For this review, take the finished solid that the model builds, in its own axes (mm). A direction names the side the tool comes from. Coordinates: 2 decimals unless noted, no trailing zeros. Order: outer loops, then holes, each group sorted by start corner. A loop starts at its lowest first (then second) coordinate and runs counter-clockwise, first axis right, second up. Notation, with made-up numbers: (89, 19) -> (99, 19) arc R8 ccw to (99, 26) -> close; hole circle Ø5 at (-29, 45). An arc over 180 degrees is marked (long way). Answer as a JSON object with one key per item and string values. Group by question number.
1) Add section B-B, the plane y = -1.5. Write out the cut boundary in (x, z), then the cut area to 3 significant figures.
2) For pin 1 (5 mm diameter, centred on x = 12, z = 1, fed in from -Y); pin 2 (1.5 mm diameter, centred on x = -4, z = 7.5, fed in from +Y); pin 3 (0.7 mm diameter, centred on y = -6, z = 2.5, fed in from +X); pin 4 (2 mm diameter, centred on x = 6.5, y = 0.5, fed in from -Z), all flat-tipped, find the tip position at first contact; note any pin that passes through.
3) Add section D-D, the plane x = 5.5. Write out the cut boundary in (y, z).
4) Add section A-A, the plane z = 2.75. Write out the cut boundary in (x, y), then the cut area to 3 significant figures.
5) Wall thickness on L1, parallel to Y at x = 5.5, z = 5.75; L2, parallel to Y at x = 0, z = 3.5; L3, parallel to X at y = 1, z = 3.75: over which ranges is each line inside the solid? List them lowest first.
6) Machinability: for faces 5 (the flat face through (-7.933, 2, 4)), 6 (the flat face through (6, -3.137, 4)), which of the approach directions +Z, -Z, +X, -X, +Y, -Y give a long, thin tool a straight path to every point of the face, cutting with its end or side? Answer none if there is none.
7) Draft analysis for pull direction X (two halves, no side actions). For faces 1 (the cylindrical face through (-0.54, -2.44, 4.44)), 2 (the flat face through (-5, -7, 4)), 3 (the flat face through (12.67, 7.07, 4.44)), 4 (the flat face through (2, 5.957, 4)), state which applies: +X half, -X half, draft (parallel to the pull), parting line (faces both ways), or undercut.
8) Add section C-C, the plane x = 0. Write out the cut boundary in (y, z), then the cut area to 3 significant figures.
from build123d import *

# Parameters (mm, degrees)
SKETCH_1_R      = 2.5
EXTRUDE_1_DEPTH = 9


with BuildPart() as part:
    # 스케치1 → 보스-돌출1 (new body)
    with BuildSketch(Plane.XY):
        with BuildLine():
            Line((-7.933325128, 1.188242905), (-5, -2.066412243))
            Line((-5, -2.066412243), (-5, -11.820871263))
            Line((-5, -11.820871263), (-3.253479839, -11.820871263))
            Line((-3.253479839, -11.820871263), (1.87605446, -7.031414053))
            Line((1.87605446, -7.031414053), (1.87605446, -4.634697365))
            ThreePointArc((1.87605446, -4.634697365), (2.980195691, -4.014776911), (3.893195608, -3.13736003))
            Line((3.893195608, -3.13736003), (9.172978659, -3.13736003))
            Line((9.172978659, -3.13736003), (14.557074242, 2.286312605))
            Line((14.557074242, 2.286312605), (14.557074242, 5.198022376))
            Line((14.557074242, 5.198022376), (10.725649804, 9.001488547))
            Line((10.725649804, 9.001488547), (6.528593017, 9.001488547))
            Line((6.528593017, 9.001488547), (6.037882178, 5.957406269))
            Line((6.037882178, 5.957406269), (-1.376355668, 5.957406269))
            Line((-1.376355668, 5.957406269), (-7.933325128, 2.286312605))
            Line((-7.933325128, 2.286312605), (-7.933325128, 1.188242905))
        make_face()
        Circle(SKETCH_1_R, mode=Mode.SUBTRACT)
    extrude(amount=EXTRUDE_1_DEPTH)


solid = part.part
Output values:
{
 "1": {"outline": "(-5.51, 0) -> (-2, 0) -> (-2, 9) -> (-5.51, 9) -> close; (2, 0) -> (10.8, 0) -> (10.8, 9) -> (2, 9) -> close", "area": "111 mm²"},
 "2": {"pin 1": "stops at y = -2.81", "pin 2": "stops at y = 4.91", "pin 3": "stops at x = 1.88", "pin 4": "stops at z = 0"},
 "3": {"outline": "(-3.14, 0) -> (5.96, 0) -> (5.96, 9) -> (-3.14, 9) -> close"},
 "4": {"outline": "(-7.93, 1.19) -> (-5, -2.07) -> (-5, -11.82) -> (-3.25, -11.82) -> (1.88, -7.03) -> (1.88, -4.63) arc R5 ccw to (3.89, -3.14) -> (9.17, -3.14) -> (14.56, 2.29) -> (14.56, 5.2) -> (10.73, 9) -> (6.53, 9) -> (6.04, 5.96) -> (-1.38, 5.96) -> (-7.93, 2.29) -> close; hole circle Ø5 at (0, 0)", "area": "217 mm²"},
 "5": {"L1": "y = -3.14 to 5.96", "L2": "y = -8.78 to -2.5, 2.5 to 5.96", "L3": "x = -7.76 to -2.29, 2.29 to 13.28"},
 "6": {"face 5": "+Z, -Z, -X, +Y, -Y", "face 6": "+Z, -Z, +X, -Y"},
 "7": {"face 1": "undercut", "face 2": "-X half", "face 3": "+X half", "face 4": "draft"},
 "8": {"outline": "(-8.78, 0) -> (-2.5, 0) -> (-2.5, 9) -> (-8.78, 9) -> close; (2.5, 0) -> (5.96, 0) -> (5.96, 9) -> (2.5, 9) -> close", "area": "87.7 mm²"}
}
